Drawing for the job (mm, zero at the part's lowest x, y, z). Give positions to 0.01 mm unless a question says otherwise; leave off trailing zeros. Order: outer loops, then holes, each group sorted by start corner. A loop starts at its lowest first (then second) coordinate and runs counter-clockwise, first axis right, second up. Notation, with made-up numbers: (29, 11.5) -> (75, 11.5) arc R9 ccw to (75, 20.5) -> close; hole circle Ø2 at (-5, 39). An arc over 180 degrees is marked (long way). Use one line per item in the form item = value. Start each with the question number.
1) Cut at A-A, the plane x = 18. Give the cut face in (y, z).
2) Mould opens along Y. For the marked faces 1, 2, 3 and 4 say: pulls with the +Y half, pulls with the -Y half, needs draft (parallel to the pull), parting line crosses it, or undercut.
3) Probe line 1 (Y direction, x = 17, z = 1); line 2 (Y direction, x = 17.75, z = 1.8); line 3 (X direction, y = 2.75, z = 0.8). List the from-to ranges inside material, lowest first.
4) Cut at C-C, the plane z = 1.75. Give the cut face in (x, y).
5) Drop a flat-ended pin along its axis: P1, Ø3, axis at x = 17, y = 17, coming from the +Z side. Give the stop position or say it passes through.
6) Cut at B-B, the plane y = 3. Give the cut face in (x, z), and give its area (3 significant figures).
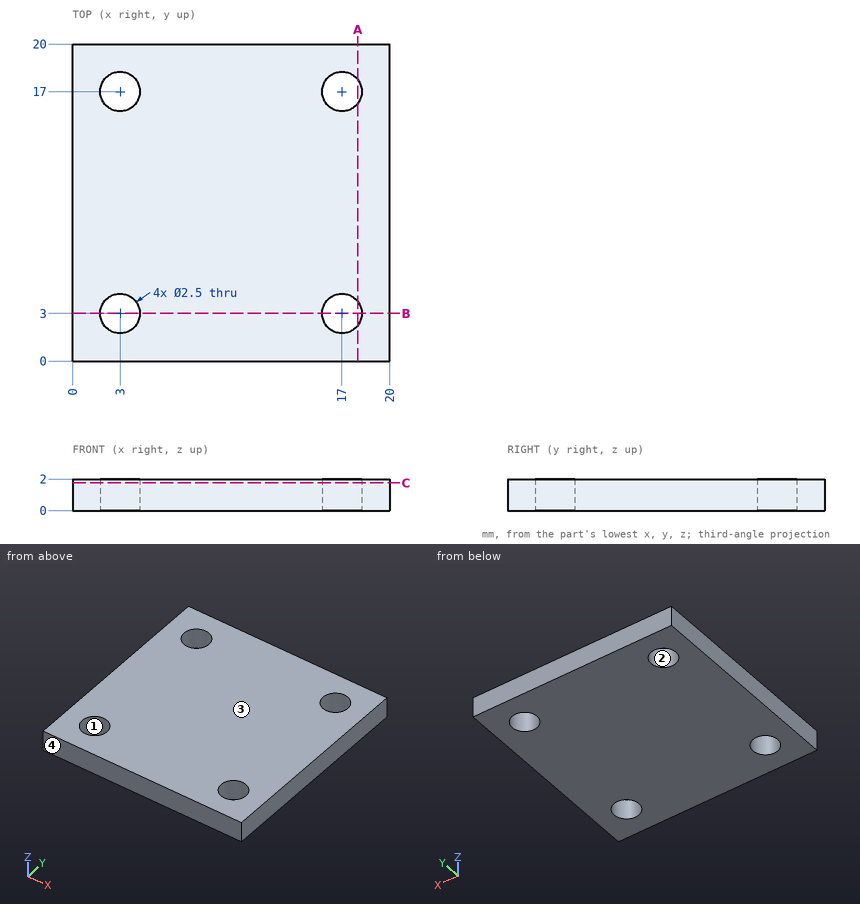
Result:
q1.outline = (0, 0) -> (2.25, 0) -> (2.25, 2) -> (0, 2) -> close; (3.75, 0) -> (16.25, 0) -> (16.25, 2) -> (3.75, 2) -> close; (17.75, 0) -> (20, 0) -> (20, 2) -> (17.75, 2) -> close
q2.face_1 = undercut
q2.face_2 = undercut
q2.face_3 = needs draft
q2.face_4 = pulls with the -Y half
q3.line_1 = 0 to 1.75, 4.25 to 15.75, 18.25 to 20
q3.line_2 = 0 to 2, 4 to 16, 18 to 20
q3.line_3 = 0 to 1.78, 4.22 to 15.78, 18.22 to 20
q4.outline = (0, 0) -> (20, 0) -> (20, 20) -> (0, 20) -> close; hole circle Ø2.5 at (3, 3); hole circle Ø2.5 at (3, 17); hole circle Ø2.5 at (17, 3); hole circle Ø2.5 at (17, 17)
q5.P1 = 2
q6.outline = (0, 0) -> (1.75, 0) -> (1.75, 2) -> (0, 2) -> close; (4.25, 0) -> (15.75, 0) -> (15.75, 2) -> (4.25, 2) -> close; (18.25, 0) -> (20, 0) -> (20, 2) -> (18.25, 2) -> close
q6.area = 30.0 mm²
